```python
from build123d import *

# Parameters (mm, degrees)
SKETCH_1_R      = 2
EXTRUDE_1_DEPTH = 312


with BuildPart() as part:
    # Sketch 1 → Extrude 1 (new body)
    with BuildSketch(Plane(origin=(0, 0, 0), x_dir=(1, 0, 0), z_dir=(0, 1, 0))):
        with BuildLine():
            Line((-10, 2.95), (-10, 9.697715604))
            ThreePointArc((-10, 9.697715604), (-9.910510619, 9.911456754), (-9.695431472, 9.997680816))
            ThreePointArc((-9.695431472, 9.997680816), (4.142135624, 4.142135624), (9.997680816, -9.695431472))
            ThreePointArc((9.997680816, -9.695431472), (9.911456754, -9.910510619), (9.697715604, -10))
            Line((9.697715604, -10), (2.95, -10))
            ThreePointArc((2.95, -10), (2.737867966, -9.912132034), (2.65, -9.7))
            Line((2.65, -9.7), (2.65, -8.8))
            ThreePointArc((2.65, -8.8), (2.737867966, -8.587867966), (2.95, -8.5))
            Line((2.95, -8.5), (3.85, -8.5))
            ThreePointArc((3.85, -8.5), (4.062132034, -8.412132034), (4.15, -8.2))
            Line((4.15, -8.2), (4.15, -4.942749448))
            ThreePointArc((4.15, -4.942749448), (4.120157221, -4.812307599), (4.03656616, -4.707817398))
            ThreePointArc((4.03656616, -4.707817398), (2.282021525, -3.714379176), (0.307277366, -3.307277366))
            Line((0.307277366, -3.307277366), (0, -3))
            Line((0, -3), (-0.307277366, -3.307277366))
            ThreePointArc((-0.307277366, -3.307277366), (-2.282021525, -3.714379176), (-4.03656616, -4.707817398))
            ThreePointArc((-4.03656616, -4.707817398), (-4.120157221, -4.812307599), (-4.15, -4.942749448))
            Line((-4.15, -4.942749448), (-4.15, -8.2))
            ThreePointArc((-4.15, -8.2), (-4.062132034, -8.412132034), (-3.85, -8.5))
            Line((-3.85, -8.5), (-2.95, -8.5))
            ThreePointArc((-2.95, -8.5), (-2.737867966, -8.587867966), (-2.65, -8.8))
            Line((-2.65, -8.8), (-2.65, -9.7))
            ThreePointArc((-2.65, -9.7), (-2.737867966, -9.912132034), (-2.95, -10))
            Line((-2.95, -10), (-9.7, -10))
            ThreePointArc((-9.7, -10), (-9.912132034, -9.912132034), (-10, -9.7))
            Line((-10, -9.7), (-10, -2.95))
            ThreePointArc((-10, -2.95), (-9.912132034, -2.737867966), (-9.7, -2.65))
            Line((-9.7, -2.65), (-8.8, -2.65))
            ThreePointArc((-8.8, -2.65), (-8.587867966, -2.737867966), (-8.5, -2.95))
            Line((-8.5, -2.95), (-8.5, -3.85))
            ThreePointArc((-8.5, -3.85), (-8.412132034, -4.062132034), (-8.2, -4.15))
            Line((-8.2, -4.15), (-4.942749448, -4.15))
            ThreePointArc((-4.942749448, -4.15), (-4.812307598, -4.120157221), (-4.707817398, -4.03656616))
            ThreePointArc((-4.707817398, -4.03656616), (-3.714379176, -2.282021525), (-3.307277366, -0.307277366))
            Line((-3.307277366, -0.307277366), (-3, 0))
            Line((-3, 0), (-3.307277366, 0.307277366))
            ThreePointArc((-3.307277366, 0.307277366), (-3.714379176, 2.282021525), (-4.707817398, 4.03656616))
            ThreePointArc((-4.707817398, 4.03656616), (-4.812307598, 4.120157221), (-4.942749448, 4.15))
            Line((-4.942749448, 4.15), (-8.2, 4.15))
            ThreePointArc((-8.2, 4.15), (-8.412132034, 4.062132034), (-8.5, 3.85))
            Line((-8.5, 3.85), (-8.5, 2.95))
            ThreePointArc((-8.5, 2.95), (-8.587867966, 2.737867966), (-8.8, 2.65))
            Line((-8.8, 2.65), (-9.7, 2.65))
            ThreePointArc((-9.7, 2.65), (-9.912132034, 2.737867966), (-10, 2.95))
        make_face()
        with Locations(Location((-7, -7, 0), (0, 0, 270))):
            Circle(SKETCH_1_R, mode=Mode.SUBTRACT)
        with BuildLine():
            Line((-5.189613301, 6.15), (-4.65, 6.15))
            ThreePointArc((-4.65, 6.15), (-4.296446609, 6.003553391), (-4.15, 5.65))
            Line((-4.15, 5.65), (-4.15, 4.942749448))
            ThreePointArc((-4.15, 4.942749448), (-4.120157221, 4.812307598), (-4.03656616, 4.707817398))
            ThreePointArc((-4.03656616, 4.707817398), (-1.420133589, 3.457261044), (1.479767066, 3.470927733))
            ThreePointArc((1.479767066, 3.470927733), (1.852984885, 3.845379716), (1.681494134, 4.345476458))
            ThreePointArc((1.681494134, 4.345476458), (-1.571941665, 6.468692501), (-5.197046609, 7.865655284))
            ThreePointArc((-5.197046609, 7.865655284), (-8.999981229, 6.991334811), (-5.189613301, 6.15))
        make_face(mode=Mode.SUBTRACT)
        with BuildLine():
            Line((6.15, -4.65), (6.15, -5.189613301))
            ThreePointArc((6.15, -5.189613301), (6.991334811, -8.999981229), (7.865655284, -5.197046609))
            ThreePointArc((7.865655284, -5.197046609), (6.468692501, -1.571941665), (4.345476458, 1.681494134))
            ThreePointArc((4.345476458, 1.681494134), (3.845379716, 1.852984885), (3.470927733, 1.479767066))
            ThreePointArc((3.470927733, 1.479767066), (3.457261044, -1.420133589), (4.707817398, -4.03656616))
            ThreePointArc((4.707817398, -4.03656616), (4.812307599, -4.120157221), (4.942749448, -4.15))
            Line((4.942749448, -4.15), (5.65, -4.15))
            ThreePointArc((5.65, -4.15), (6.003553391, -4.296446609), (6.15, -4.65))
        make_face(mode=Mode.SUBTRACT)
        with BuildLine():
            Line((-2.257496667, -1.550389886), (-1.99100568, -1.283898899))
            ThreePointArc((-1.99100568, -1.283898899), (-1.907277277, -1.121431759), (-1.933365749, -0.940530106))
            ThreePointArc((-1.933365749, -0.940530106), (-2.15, 0), (-1.933365749, 0.940530106))
            ThreePointArc((-1.933365749, 0.940530106), (-1.907277277, 1.121431759), (-1.99100568, 1.283898899))
            Line((-1.99100568, 1.283898899), (-2.257496667, 1.550389886))
            ThreePointArc((-2.257496667, 1.550389886), (-2.345158518, 1.75140317), (-2.27262737, 1.958357689))
            ThreePointArc((-2.27262737, 1.958357689), (-2.121320344, 2.121320344), (-1.958357689, 2.27262737))
            ThreePointArc((-1.958357689, 2.27262737), (-1.75140317, 2.345158518), (-1.550389886, 2.257496667))
            Line((-1.550389886, 2.257496667), (-1.283898899, 1.99100568))
            ThreePointArc((-1.283898899, 1.99100568), (-1.121431759, 1.907277277), (-0.940530106, 1.933365749))
            ThreePointArc((-0.940530106, 1.933365749), (0, 2.15), (0.940530106, 1.933365749))
            ThreePointArc((0.940530106, 1.933365749), (1.12143176, 1.907277277), (1.283898899, 1.99100568))
            Line((1.283898899, 1.99100568), (1.550389886, 2.257496667))
            ThreePointArc((1.550389886, 2.257496667), (1.75140317, 2.345158518), (1.958357689, 2.27262737))
            ThreePointArc((1.958357689, 2.27262737), (2.121320344, 2.121320344), (2.27262737, 1.958357689))
            ThreePointArc((2.27262737, 1.958357689), (2.345158518, 1.75140317), (2.257496667, 1.550389886))
            Line((2.257496667, 1.550389886), (1.99100568, 1.283898899))
            ThreePointArc((1.99100568, 1.283898899), (1.907277277, 1.121431759), (1.933365749, 0.940530105))
            ThreePointArc((1.933365749, 0.940530105), (2.15, 0), (1.933365749, -0.940530106))
            ThreePointArc((1.933365749, -0.940530106), (1.907277277, -1.121431759), (1.99100568, -1.283898899))
            Line((1.99100568, -1.283898899), (2.257496667, -1.550389886))
            ThreePointArc((2.257496667, -1.550389886), (2.345158518, -1.75140317), (2.27262737, -1.958357689))
            ThreePointArc((2.27262737, -1.958357689), (2.121320344, -2.121320344), (1.958357689, -2.27262737))
            ThreePointArc((1.958357689, -2.27262737), (1.75140317, -2.345158518), (1.550389886, -2.257496667))
            Line((1.550389886, -2.257496667), (1.283898899, -1.99100568))
            ThreePointArc((1.283898899, -1.99100568), (1.121431759, -1.907277277), (0.940530106, -1.933365749))
            ThreePointArc((0.940530106, -1.933365749), (0, -2.15), (-0.940530105, -1.933365749))
            ThreePointArc((-0.940530105, -1.933365749), (-1.121431759, -1.907277277), (-1.283898899, -1.99100568))
            Line((-1.283898899, -1.99100568), (-1.550389886, -2.257496667))
            ThreePointArc((-1.550389886, -2.257496667), (-1.75140317, -2.345158518), (-1.958357689, -2.27262737))
            ThreePointArc((-1.958357689, -2.27262737), (-2.121320344, -2.121320344), (-2.27262737, -1.958357689))
            ThreePointArc((-2.27262737, -1.958357689), (-2.345158518, -1.75140317), (-2.257496667, -1.550389886))
        make_face(mode=Mode.SUBTRACT)
    extrude(amount=EXTRUDE_1_DEPTH)


solid = part.part
```
For this review, take the finished solid that the model builds, in its own axes (mm). A direction names the side the tool comes from. Give positions to 0.01 mm unless a question says otherwise; leave off trailing zeros.
Item 1: Wall thickness on probe 1 along X at (y, z) = (227, 7); probe 2 along Z at (x, y) = (-8.25, 67); probe 3 along Z at (x, y) = (5.25, 266.5): over which ranges is each line inside the solid? List them lowest first.
Item 2: The part is to be moulded in two halves that separate along Z. For faces 3 (the face through (3.99, 153.82, -4.29)), 4 (the face through (6, 154, 10)), 5 (the face through (-1.46, 153.816, -3.466)), 6 (the face through (-3, 0, 1)), say which applies: +Z half, -Z half, draft (parallel to the pull), parting line (faces both ways), or undercut.
Item 3: Take a section at A-A (y = 49.5). Give the number of separate pieces and of enclosed holes in the cut face, and give its area (3 significant figures).
Item 4: Insertion check: P1, Ø6, axis at x = -6, y = 109, coming from the -Z side (3 decimals); P2, Ø1, axis at y = 96.5, z = -3.5, coming from the +X side; P3, Ø2.5, axis at y = 185.5, z = 6.5, coming from the +X side. Each pin has a flat end and moves straight along its axis. Give the tip position at first contact, or say it passes through.
Item 5: Machinability: for faces 1 (the face through (-6, 154, 10)), 2 (the face through (6.493, 153.816, 1.62)), which of the approach directions +Z, -Z, +X, -X, +Y, -Y give a long, thin tool a straight path to every point of the face, cutting with its end or side? Answer none if there is none.
Established:
1. probe 1: x = -10 to -9, -5 to -4.15, 4.15 to 5, 9 to 9.77
1. probe 2: z = -9.92 to -8.56, -5.44 to -4.15, 4.15 to 5.44, 8.56 to 10
1. probe 3: z = -2.94 to -0.47, 4.15 to 6.03, 7.97 to 10
2. face 3: -Z half
2. face 4: +Z half
2. face 5: undercut
2. face 6: draft
3. separate pieces: 1
3. enclosed holes: 4
3. area: 131 mm2
4. P1: stops at z = -9.975
4. P2: stops at x = 5.2
4. P3: stops at x = 9.87
5. face 1: +Z, +X, -X, +Y, -Y
5. face 2: +Y, -Y
